from build123d import *

# Parameters (mm, degrees)
F0_R     = 2
F0_R_2   = 2.65
F1_DEPTH = 10


with BuildPart() as f1:
    # F0 (on Top) → F1 (new body)
    with BuildSketch(Plane.XY):
        with BuildLine():
            Line((-5.035349, -10.106315), (56.964651, -10.106315))
            ThreePointArc((56.964651, -10.106315), (60.500185, -8.641849), (61.964651, -5.106315))
            Line((61.964651, -5.106315), (61.964651, 29.291359))
            ThreePointArc((61.964651, 29.291359), (61.726129, 30.817247), (61.033319, 32.19755))
            Line((61.033319, 32.19755), (39.888801, 61.799876))
            ThreePointArc((39.888801, 61.799876), (38.108041, 63.339523), (35.820133, 63.893685))
            Line((35.820133, 63.893685), (-5.035349, 63.893685))
            ThreePointArc((-5.035349, 63.893685), (-8.570883, 62.429219), (-10.035349, 58.893685))
            Line((-10.035349, 58.893685), (-10.035349, 56.893685))
            ThreePointArc((-10.035349, 56.893685), (-8.570883, 53.358151), (-5.035349, 51.893685))
            Line((-5.035349, 51.893685), (28.391562, 51.893685))
            ThreePointArc((28.391562, 51.893685), (30.67947, 51.339523), (32.460229, 49.799876))
            Line((32.460229, 49.799876), (45.033319, 32.19755))
            ThreePointArc((45.033319, 32.19755), (45.726129, 30.817247), (45.964651, 29.291359))
            Line((45.964651, 29.291359), (45.964651, 6.893685))
            ThreePointArc((45.964651, 6.893685), (44.500185, 3.358151), (40.964651, 1.893685))
            Line((40.964651, 1.893685), (-5.035349, 1.893685))
            ThreePointArc((-5.035349, 1.893685), (-8.570883, 0.429219), (-10.035349, -3.106315))
            Line((-10.035349, -3.106315), (-10.035349, -5.106315))
            ThreePointArc((-10.035349, -5.106315), (-8.570883, -8.641849), (-5.035349, -10.106315))
        make_face()
        with Locations((-4.035349, -4.106315)):
            Circle(F0_R, mode=Mode.SUBTRACT)
        with Locations((18.964651, -4.106315)):
            Circle(F0_R, mode=Mode.SUBTRACT)
        with Locations((53.964651, -4.106315)):
            Circle(F0_R_2, mode=Mode.SUBTRACT)
        with BuildLine():
            ThreePointArc((49.964651, 20.893685), (50.843331, 23.015005), (52.964651, 23.893685))
            Line((52.964651, 23.893685), (54.964651, 23.893685))
            ThreePointArc((54.964651, 23.893685), (57.085972, 23.015005), (57.964651, 20.893685))
            Line((57.964651, 20.893685), (57.964651, 4.893685))
            ThreePointArc((57.964651, 4.893685), (57.085972, 2.772364), (54.964651, 1.893685))
            Line((54.964651, 1.893685), (52.964651, 1.893685))
            ThreePointArc((52.964651, 1.893685), (50.843331, 2.772364), (49.964651, 4.893685))
            Line((49.964651, 4.893685), (49.964651, 20.893685))
        make_face(mode=Mode.SUBTRACT)
        with Locations((-4.035349, 57.893685)):
            Circle(F0_R, mode=Mode.SUBTRACT)
        with Locations((18.964651, 57.893685)):
            Circle(F0_R, mode=Mode.SUBTRACT)
        with Locations((53.964651, 29.893685)):
            Circle(F0_R_2, mode=Mode.SUBTRACT)
    extrude(amount=F1_DEPTH)


solid = f1.part
Design review of the part built by this model. Coordinates are the model's own, in mm. A direction names the side the tool comes from. Round coordinates to 2 decimals unless told otherwise and drop trailing zeros. Write each loop counter-clockwise with the first axis right and the second up, starting at its lowest first coordinate (ties: lowest second). Pieces come first, ordered by that corner, then holes. Notation, with made-up numbers: (34, 65.5) -> (66, 65.5) arc R29 cw to (66, 92.5) -> close; hole circle Ø9 at (-4.75, 73). An arc over 180 degrees is marked (long way). One line per question, with ' | ' between items.
(1) Take a section at B-B, the plane y = 12.5. State the section outline as (x, z) points.
Result sheet:
outline: (45.96, 0) -> (49.96, 0) -> (49.96, 10) -> (45.96, 10) -> close; (57.96, 0) -> (61.96, 0) -> (61.96, 10) -> (57.96, 10) -> close
(2) Take a section at D-D, the plane z = 2.5. State how many separate pieces and enclosed holes the cut face has, and give its area (3 significant figures).
Result sheet:
separate pieces: 1 | enclosed holes: 7 | area: 2,010 mm2
(3) Take a section at C-C, the plane x = 54. State the section outline as (y, z) points, and give its area (3 significant figures).
Result sheet:
outline: (-10.11, 0) -> (-6.76, 0) -> (-6.76, 10) -> (-10.11, 10) -> close; (-1.46, 0) -> (1.89, 0) -> (1.89, 10) -> (-1.46, 10) -> close; (23.89, 0) -> (27.24, 0) -> (27.24, 10) -> (23.89, 10) -> close; (32.54, 0) -> (42.04, 0) -> (42.04, 10) -> (32.54, 10) -> close | area: 196 mm2
(4) Insertion check: P1, Ø2, axis at x = 54, z = 4.5, coming from the +Y side; P2, Ø5, axis at x = 18.96, y = -4.11, coming from the +Z side; P3, Ø1.5, axis at x = 41, z = 8.5, coming from the +Y side; P4, Ø5, axis at y = 9, z = 3.5, coming from the -X side. Each pin has a flat end and moves straight along its axis. Give the tip position at first contact, or say it passes through.
Result sheet:
P1: y = 43.44 | P2: z = 10 | P3: y = 61.29 | P4: x = 45.95
(5) Take a section at A-A, the plane x = 0. State the section outline as (y, z) points, and give its area (3 significant figures).
Result sheet:
outline: (-10.11, 0) -> (1.89, 0) -> (1.89, 10) -> (-10.11, 10) -> close; (51.89, 0) -> (63.89, 0) -> (63.89, 10) -> (51.89, 10) -> close | area: 240 mm2
(6) Draft analysis for pull direction X (two halves, no side actions). For faces 1 (the cylindrical face through (61.73, 30.8, 4.93)), 2 (the flat face through (18, 1.894, 5)), 3 (the cylindrical face through (-4.296, 59.877, 4.93)), 4 (the cylindrical face through (-8.61, 53.4, 4.93)), state which applies: released by +X, released by -X, zero draft, split by the parting line, or undercut.
Result sheet:
face 1: released by +X | face 2: zero draft | face 3: undercut | face 4: released by -X
(7) Wall thickness on line 1 (Y direction, x = 19, z = 9.25); line 2 (Y direction, x = 4, z = 2.75); line 3 (X direction, y = 12, z = 8): over which ranges is each line inside the solid? List them lowest first. Write a range as [from, to].
Result sheet:
line 1: [-10.11, -6.11], [-2.11, 1.89], [51.89, 55.89], [59.89, 63.89] | line 2: [-10.11, 1.89], [51.89, 63.89] | line 3: [45.96, 49.96], [57.96, 61.96]
(8) Machinability: for faces 5 (the cylindrical face through (-8.5, 0.5, 4.9)), 6 (the cylindrical face through (60.46, -8.68, 4.93)), 7 (the cylindrical face through (50.82, 22.99, 4.93)), which of the approach directions +Z, -Z, +X, -X, +Y, -Y give a long, thin tool a straight path to every point of the face, cutting with its end or side? Answer none if there is none.
Result sheet:
face 5: +Z, -Z, -X | face 6: +Z, -Z, +X, -Y | face 7: +Z, -Z
